The model under review builds one solid part; all positions refer to its coordinate system, in mm. A direction names the side the tool comes from. Coordinates: 2 decimals unless noted, no trailing zeros. Loops run counter-clockwise (first coordinate to the right, second up) from the corner with the lowest first, then second, coordinate; pieces in that order, holes last. Notation, with made-up numbers: M -25.5,-5.75 L 8.5,-5.75 A6 cw 8.5,5.25 Z; hole C 34,-1.75 d3. An arc over 180 degrees is marked long. Use CSV: the item, a comma, the result in double quotes. Start each with the question number.
1. Tool access review of faces 1 (the cylindrical face through (55.26, 6.1, 3.55)), 2 (the cylindrical face through (44.747, 11.264, 3.549)), 3 (the cylindrical face through (44.747, -0.264, 3.549)): name each direction out of +Z, -Z, +X, -X, +Y, -Y from which nothing blocks a thin tool from reaching the whole face with its end or side.
2. Add section A-A, the plane x = 4. Write out the cut boundary in (y, z).
3. Add section C-C, the plane z = 3. Write out the cut boundary in (x, y), then the cut area to 3 significant figures.
4. Clearance check with flat-ended pins moving along their axes: P1, Ø3, axis at x = 46.5, z = 1.5, coming from the -Y side; P2, Ø2, axis at y = -1, z = 3, coming from the +X side; P3, Ø2, axis at x = 46.5, y = 4, coming from the -Z side; P4, Ø2, axis at x = 59.14, y = 9.44, coming from the +Z side. State where each tip first meets the part, or that it passes through.
5. Add section B-B, the plane y = 5.5. Write out the cut boundary in (x, z), then the cut area to 3 significant figures.
6. Draft analysis for pull direction X (two halves, no side actions). For faces 4 (the flat face through (4, 8, -1)), 5 (the cylindrical face through (46.042, 2.038, 3.451)), state which applies: +X half, -X half, draft (parallel to the pull), parting line (faces both ways), or undercut.
7. Add section D-D, the plane y = 10.25. Write out the cut boundary in (x, z).
8. For L1, parallel to Z at x = 4, y = 12.5; L2, parallel to X at y = 0.75, z = 0.75; L3, parallel to Y at x = 4, z = 1, list the stretches that pass through material, from the lowest coordinate up.
from build123d import *

# Parameters (mm, degrees)
BOSS_EXTRUDE1_DEPTH      = 7
SKETCH2_R                = 2
CUT_EXTRUDE1_DEPTH       = 66.594825405
FILLET11_R               = 3
SKETCH32_R               = 2
CUT_EXTRUDE14_DEPTH      = 66.594825405
SKETCH33_R               = 9
SKETCH33_R_2             = 2
BOSS_EXTRUDE2_DEPTH      = 8
SKETCH35_R               = 1.6
SKETCH35_R_2             = 1.75
CUT_EXTRUDE15_DEPTH      = 66.594825405
CUT_EXTRUDE16_DEPTH      = 65.51690569
CUT_EXTRUDE16_DEPTH_BACK = 65.51690569
SKETCH37_R               = 1.51


with BuildPart() as part:
    # Sketch1 → Boss-Extrude1 (new body)
    with BuildSketch(Plane.XY):
        with BuildLine():
            Line((0, 11), (0, 0))
            Line((0, 0), (45, 0))
            ThreePointArc((45, 0), (63.351646544, 5.5), (45, 11))
            Line((45, 11), (0, 11))
        make_face()
    extrude(amount=BOSS_EXTRUDE1_DEPTH)

    # Sketch2 → Cut-Extrude1 (cut, through all)
    with BuildSketch(Plane.XY.offset(7)):
        with Locations((53.351646544, 5.5)):
            Circle(SKETCH2_R)
        with Locations((-8.351646544, 5.5)):
            Circle(SKETCH2_R)
    extrude(amount=-CUT_EXTRUDE1_DEPTH, mode=Mode.SUBTRACT)

    # Fillet11
    fillet11_edges = [part.edges().sort_by_distance(p)[0] for p in [
        (45, 11, 3.5),
        (45, 0, 3.5),
    ]]
    fillet(fillet11_edges, radius=FILLET11_R)

    # Sketch32 → Cut-Extrude14 (cut, through all)
    with BuildSketch(Plane.XY.offset(7)):
        with Locations((4, 5.5)):
            Circle(SKETCH32_R)
    extrude(amount=-CUT_EXTRUDE14_DEPTH, mode=Mode.SUBTRACT)

    # Sketch33 → Boss-Extrude2 (add)
    with BuildSketch(Plane.XY.offset(7)):
        with Locations((4, 5.5)):
            Circle(SKETCH33_R)
        with Locations((4, 5.5)):
            Circle(SKETCH33_R_2, mode=Mode.SUBTRACT)
    extrude(amount=-BOSS_EXTRUDE2_DEPTH)

    # Sketch35 → Cut-Extrude15 (cut, through all)
    with BuildSketch(Plane(origin=(0, 0, 0), x_dir=(-1, 0, 0), z_dir=(0, 0, -1))):
        with Locations((-47.567725348, 1.557125972)):
            Circle(SKETCH35_R)
        with Locations((-57.294520572, -0.283921196)):
            Circle(SKETCH35_R_2)
        with Locations((-59.13556774, 9.442874028)):
            Circle(SKETCH35_R_2)
        with Locations((-49.408772516, 11.283921196)):
            Circle(SKETCH35_R_2)
    extrude(amount=-CUT_EXTRUDE15_DEPTH, mode=Mode.SUBTRACT)

    # Sketch37 → Cut-Extrude16 (cut, two sides: drawn at the far end of the back side and taken through both)
    with BuildSketch(Plane(origin=(0, 5.5, 0), x_dir=(1, 0, 0), z_dir=(0, 1, 0)).offset(-CUT_EXTRUDE16_DEPTH_BACK)):
        with Locations(Location((4, -3, 0), (0, 0, 270))):
            Circle(SKETCH37_R)
    extrude(amount=CUT_EXTRUDE16_DEPTH + CUT_EXTRUDE16_DEPTH_BACK, mode=Mode.SUBTRACT)


solid = part.part
Computed:
1,face 1,"+Z, -Z"
1,face 2,"+Z, -Z, +Y"
1,face 3,"+Z, -Z, -Y"
2,outline,"M -3.5,-1 L 3.5,-1 L 3.5,1.49 L -3.5,1.49 Z; M -3.5,4.51 L 3.5,4.51 L 3.5,7 L -3.5,7 Z; M 7.5,-1 L 14.5,-1 L 14.5,1.49 L 7.5,1.49 Z; M 7.5,4.51 L 14.5,4.51 L 14.5,7 L 7.5,7 Z"
3,outline,"M 2.49,-3.37 L 2.49,4.19 A2 cw 2.49,6.81 L 2.49,14.37 A9 ccw Z; M 5.51,-3.37 A9 ccw 11.12,0 L 43.52,0 A3 cw 45.79,-1.04 A10 ccw long 45.79,12.04 A3 cw 43.52,11 L 11.12,11 A9 ccw 5.51,14.37 L 5.51,6.81 A2 cw 5.51,4.19 Z; hole C 47.57,1.56 d3.2; hole C 49.41,11.28 d3.5; hole C 53.35,5.5 d4; hole C 57.29,-0.28 d3.5; hole C 59.14,9.44 d3.5"
3,area,"810 mm^2"
4,P1,"stops at y = -2.95"
4,P2,"stops at x = 61.7"
4,P3,"stops at z = 0"
4,P4,"passes through"
5,outline,"M -5,-1 L 2,-1 L 2,7 L -5,7 Z; M 6,-1 L 13,-1 L 13,0 L 51.35,0 L 51.35,7 L 6,7 Z; M 55.35,0 L 63.35,0 L 63.35,7 L 55.35,7 Z"
5,area,"436 mm^2"
6,face 4,"draft"
6,face 5,"undercut"
7,outline,"M -3.64,-1 L 11.64,-1 L 11.64,0 L 48,0 L 48,7 L -3.64,7 Z; M 50.82,0 L 57.58,0 L 57.58,7 L 50.82,7 Z; M 60.69,0 L 62.15,0 L 62.15,7 L 60.69,7 Z; hole C 4,3 d3.02"
8,L1,"z = -1 to 1.49, 4.51 to 7"
8,L2,"x = -3.64 to 46.19, 48.95 to 55.88, 58.71 to 62.15"
8,L3,"y = -3.5 to 3.5, 7.5 to 14.5"
